Part print with two shaded views. Sizes in mm from the minimum x, y, z corner. A direction names the side the tool comes from. Round coordinates to 2 decimals unless told otherwise and drop trailing zeros. Loops run counter-clockwise (first coordinate to the right, second up) from the corner with the lowest first, then second, coordinate; pieces in that order, holes last.
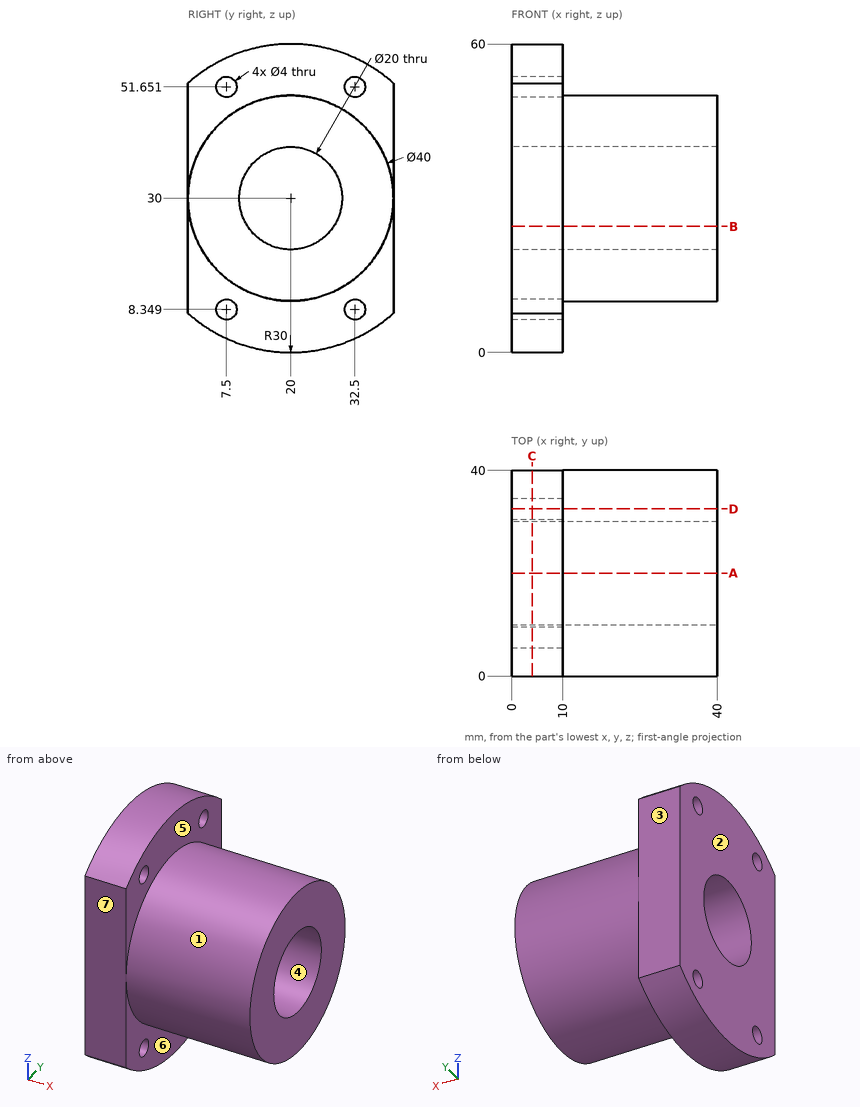
Item 1: Cut at C-C (x = 4). List the corners of the cut face in (y, z).
Verdict:
outline: (0, 7.64) arc R30 ccw to (40, 7.64) - (40, 52.36) arc R30 ccw to (0, 52.36) - close; hole circle Ø4 at (7.5, 8.35); hole circle Ø4 at (7.5, 51.65); hole circle Ø20 at (20, 30); hole circle Ø4 at (32.5, 8.35); hole circle Ø4 at (32.5, 51.65)
Item 2: Wall check: L1, parallel to Z at x = 3.75, y = 7.5; L2, parallel to Z at x = 2, y = 32 (1 decimal); L3, parallel to X at y = 19, z = 55. Give the ranges that are in metal, low to high.
Verdict:
L1: z = 2.73 to 6.35, 10.35 to 49.65, 53.65 to 57.27
L2: z = 2.5 to 6.4, 10.3 to 49.7, 53.6 to 57.5
L3: x = 0 to 10
Item 3: 3-axis set-ups, long thin cutter, end or side, ignore diameter. For the marked faces 5, 6 and 7: which of +Z, -Z, +X, -X, +Y, -Y reach the whole face in a straight line?
Verdict:
face 5: +Z, +X
face 6: -Z, +X
face 7: +Z, -Z, +X, -X, -Y
Item 4: Flat gauge pins, fed straight in: P1, Ø4.5, axis at y = 7.5, z = 51.65, coming from the +X side; P2, Ø1, axis at x = 21, y = 5, coming from the +Z side (1 decimal); P3, Ø10, axis at x = 24.5, z = 10.5, coming from the +Y side (1 decimal); P4, Ø4, axis at x = 4.5, z = 53, coming from the +Y side. Where does each tip first touch, or does it go through?
Verdict:
P1: stops at x = 10
P2: stops at z = 43.8
P3: stops at y = 33.8
P4: stops at y = 40
Item 5: Mould opens along Y. For the marked faces 1, 2, 3 and 4 say: released by +Y, released by -Y, zero draft, split by the parting line, or undercut.
Verdict:
face 1: split by the parting line
face 2: zero draft
face 3: released by +Y
face 4: undercut
Item 6: Cut at A-A (y = 20). List the corners of the cut face in (x, z), plus the area to 3 significant figures.
Verdict:
outline: (0, 0) - (10, 0) - (10, 10) - (40, 10) - (40, 20) - (0, 20) - close; (0, 40) - (40, 40) - (40, 50) - (10, 50) - (10, 60) - (0, 60) - close
area: 1,000 mm2
Item 7: Cut at B-B (z = 24.5). List the corners of the cut face in (x, y).
Verdict:
outline: (0, 0) - (10, 0) - (10, 0.77) - (40, 0.77) - (40, 11.65) - (0, 11.65) - close; (0, 28.35) - (40, 28.35) - (40, 39.23) - (10, 39.23) - (10, 40) - (0, 40) - close
Item 8: Cut at D-D (y = 32.5). List the corners of the cut face in (x, z).
Verdict:
outline: (0, 2.73) - (10, 2.73) - (10, 6.35) - (0, 6.35) - close; (0, 10.35) - (10, 10.35) - (10, 14.39) - (40, 14.39) - (40, 45.61) - (10, 45.61) - (10, 49.65) - (0, 49.65) - close; (0, 53.65) - (10, 53.65) - (10, 57.27) - (0, 57.27) - close
